Here's how the part is built. I have some questions about the finished solid (model axes, mm). Face numbers are marked on the shaded views. A direction names the side the tool comes from. Give positions to 0.01 mm unless a question says otherwise; leave off trailing zeros. Order: outer loops, then holes, each group sorted by start corner. A loop starts at its lowest first (then second) coordinate and runs counter-clockwise, first axis right, second up.
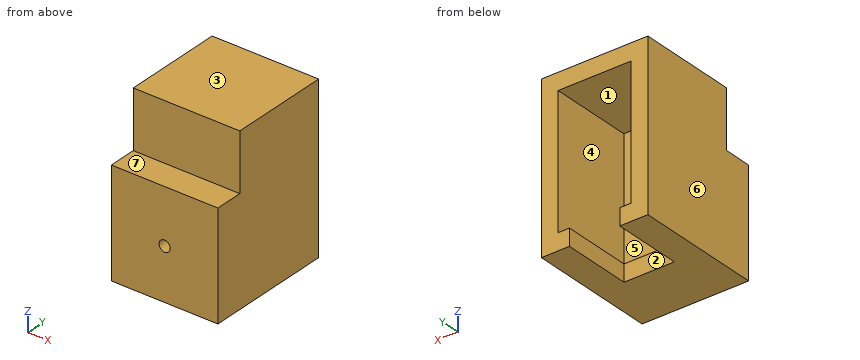
Autodesk Inventor part; units mm, degrees
ref_plane "YZ Plane" through (0, 0, 0) normal (1, 0, 0) x (0, 1, 0)
ref_plane "XZ Plane" through (0, 0, 0) normal (0, 1, 0) x (-1, 0, 0)
ref_plane "XY Plane" through (0, 0, 0) normal (0, 0, 1) x (1, 0, 0)
sketch "Sketch1" plane through (0, 0, 0) normal (0, 1, 0) x (-1, 0, 0)
  line L0 (6.225, 11.375) -> (-6.225, 11.375)
  line L1 (-6.225, 11.375) -> (-6.225, -11.375)
  line L2 (-6.225, -11.375) -> (6.225, -11.375)
  line L3 (6.225, -11.375) -> (6.225, 11.375)
  line L4 (6.225, 11.375) -> (-6.225, -11.375) construction
  line L5 (-6.225, 11.375) -> (6.225, -11.375) construction
  line L6 (9.525, 14.675) -> (-9.525, 14.675)
  line L7 (-9.525, 14.675) -> (-9.525, -14.675)
  line L8 (-9.525, -14.675) -> (9.525, -14.675)
  line L9 (9.525, -14.675) -> (9.525, 14.675)
  point P0 (0, 0)
  dimension "d0" = 12.45
  dimension "d1" = 22.75
  dimension "d2" = 3.3
extrude "Extrusion1" add sketch "Sketch1" along normal blind 15
sketch "Sketch2" plane through (9.525, 0, -14.675) normal (0, 0, -1) x (-1, 0, 0)
  line L0 (14.025, 2.55) -> (5.025, 2.55)
  line L1 (5.025, 2.55) -> (5.025, 6.55)
  line L2 (14.025, 6.55) -> (14.025, 2.55)
  line L3 (3.3, 15) -> (15.75, 15)
  line L4 (5.025, 2.55) -> (14.025, 2.55)
  line L5 (14.025, 2.55) -> (14.025, 15)
  line L6 (14.025, 15) -> (5.025, 15)
  line L7 (5.025, 15) -> (5.025, 2.55)
  point P0 (9.525, 0)
  dimension "d7" = 9
  dimension "d8" = 4
extrude "Extrusion2" cut sketch "Sketch2" against normal up to next
sketch "Sketch3" plane through (0, 0, 0) normal (0, -1, 0) x (1, 0, 0)
  line L0 (-9.525, 14.675) -> (9.525, 14.675)
  line L1 (-9.525, -14.675) -> (-9.525, 14.675)
  line L2 (9.525, -14.675) -> (-9.525, -14.675)
  line L3 (9.525, 14.675) -> (9.525, -14.675)
  point P0 (0, 0)
extrude "Extrusion3" add sketch "Sketch3" along normal blind 3
sketch "Sketch4" plane through (0, -3, 0) normal (0, -1, 0) x (1, 0, 0)
  line L0 (6.225, 11.375) -> (6.225, -11.375)
  line L1 (6.225, -11.375) -> (-6.225, -11.375)
  line L2 (-6.225, -11.375) -> (-6.225, 11.375)
  line L3 (4.5, -11.375) -> (-4.5, -11.375)
  line L4 (0, -11.375) -> (0, -5.425)
  circle A0 centre (0, -5.425) radius 1
  point P0 (0, 0)
  dimension "d13" = 5.95
  dimension "d14" = 2
extrude "Extrusion4" cut sketch "Sketch4" against normal up to next
sketch "Sketch5" plane through (0, -3, 0) normal (0, -1, 0) x (1, 0, 0)
  circle A0 centre (0, -5.425) radius 1
  line L0 (-9.525, -14.675) -> (9.525, -14.675)
  line L1 (9.525, -14.675) -> (9.525, 4.375)
  line L2 (9.525, 4.375) -> (-9.525, 4.375)
  line L3 (-9.525, 4.375) -> (-9.525, -14.675)
  line L4 (-9.525, -14.675) -> (9.525, -14.675)
  line L5 (9.525, -14.675) -> (9.525, 4.375)
  point P0 (0, 0)
  dimension "d17" = 19.05
extrude "Extrusion5" add sketch "Sketch5" along normal blind 5
sketch "Sketch6" plane through (0, 15, 0) normal (0, 1, 0) x (1, 0, 0)
  circle A0 centre (0, 5.425) radius 1
  line L0 (-6.225, -11.375) -> (6.225, -11.375)
  line L1 (6.225, -11.375) -> (6.225, 11.375)
  line L2 (6.225, 11.375) -> (-6.225, 11.375)
  line L3 (-6.225, 11.375) -> (-6.225, -11.375)
  line L4 (0, 11.375) -> (0, 11.675)
  line L5 (-6.525, 11.675) -> (6.525, 11.675)
  line L6 (6.525, 11.675) -> (6.525, -11.675)
  line L7 (6.525, -11.675) -> (-6.525, -11.675)
  line L8 (-6.525, -11.675) -> (-6.525, 11.675)
  point P0 (0, 0)
  dimension "d20" = 0.3
extrude "Extrusion6" cut sketch "Sketch6" against normal up to surface (15 mm away) contours L3 L2 L1 L0 | L5 L6 L7 L8
properties part number "servo housing"
Q1. If we section it at D-D on x = 3: List the corners of the cut face in (y, z) for me (3 decimals), plus the area to 3 significant figures.
Filled sheet:
outline: (-8, -14.675) - (2.55, -14.675) - (2.55, -11.675) - (0, -11.675) - (0, 11.675) - (15, 11.675) - (15, 14.675) - (-3, 14.675) - (-3, 4.375) - (-8, 4.375) - close
area: 236 mm2
Q2. Thinking about a two-plate mould opening in Z: for the marked faces 1, 2, 3 and 4, which applies, released by +Z, released by -Z, zero draft, split by the parting line, or undercut?
Filled sheet:
face 1: undercut
face 2: zero draft
face 3: released by +Z
face 4: undercut
Q3. For the marked faces 5, 6 and 7, which set-ups out of +Z, -Z, +X, -X, +Y, -Y let a thin tool reach every point of the face, with its end or its side?
Filled sheet:
face 5: +Y
face 6: +Z, -Z, -X, +Y, -Y
face 7: +Z, +X, -X, -Y
Q4. I need wall thicknesses on L1, parallel to Z at x = 5, y = 8.5 (3 decimals); L2, parallel to X at y = 4.5, z = -6.25 (3 decimals); L3, parallel to Z at x = 0, y = -3.75 (3 decimals). Which ranges of each line are inside material? Lowest first, please.
Filled sheet:
L1: z = -14.675 to -11.675, 11.675 to 14.675
L2: x = -9.525 to -6.525, 6.525 to 9.525
L3: z = -14.675 to -6.425, -4.425 to 4.375
Q5. If we section it at C-C on y = 4: List the corners of the cut face in (x, z) for me (3 decimals).
Filled sheet:
outline: (-9.525, -14.675) - (-4.5, -14.675) - (-4.5, -11.675) - (-6.525, -11.675) - (-6.525, 11.675) - (6.525, 11.675) - (6.525, -11.675) - (4.5, -11.675) - (4.5, -14.675) - (9.525, -14.675) - (9.525, 14.675) - (-9.525, 14.675) - close
Q6. If we section it at A-A on x = 0: List the corners of the cut face in (y, z) for me (3 decimals).
Filled sheet:
outline: (-8, -14.675) - (2.55, -14.675) - (2.55, -11.675) - (0, -11.675) - (0, -6.425) - (-8, -6.425) - close; (-8, -4.425) - (0, -4.425) - (0, 11.675) - (15, 11.675) - (15, 14.675) - (-3, 14.675) - (-3, 4.375) - (-8, 4.375) - close
Q7. I'm going to push a flat-ended pin straight in: P1, Ø2.5, axis at x = -1, z = -13.5, coming from the +Y side. Where does the tip first touch, or does it pass through?
Filled sheet:
P1: stops at y = 2.55
Q8. If we section it at B-B on z = -12.5: List the corners of the cut face in (x, y) for me (3 decimals), plus the area to 3 significant figures.
Filled sheet:
outline: (-9.525, -8) - (9.525, -8) - (9.525, 15) - (4.5, 15) - (4.5, 2.55) - (-4.5, 2.55) - (-4.5, 15) - (-9.525, 15) - close
area: 326 mm2
